Build history of the part. All positions in model axes, mm. Round coordinates to 2 decimals unless told otherwise and drop trailing zeros. Loops run counter-clockwise (first coordinate to the right, second up) from the corner with the lowest first, then second, coordinate; pieces in that order, holes last. Notation, with made-up numbers: (22.5, -0.75) - (33.5, -0.75) arc R29 ccw to (33.5, 31.25) - close; hole circle Ø10 at (0, 82.5). An arc over 180 degrees is marked (long way). Use one line per item in the form item = value. Start each with the question number.
Q1. Saw through at C-C (y = 8.5). Give the cut face in (x, z).
Q2. Saw through at D-D (z = -13). Give the cut face in (x, y).
Q3. Saw through at A-A (z = 0). Give the cut face in (x, y).
Q4. Pin check, flat tips, straight feed: pin 1 (1.4 mm diameter, centred on x = -2, z = 13, fed in from -Y); pin 2 (1.5 mm diameter, centred on x = -1, y = 42, fed in from +Z); pin 3 (1.5 mm diameter, centred on x = -2, z = -10, fed in from +Y). Stop position of each tip, or through.
Q5. Drill centre lines: line 1 (Z direction, x = -2.25, y = 0); line 2 (Y direction, x = -2.3, z = -0.5); line 3 (Y direction, x = -0.8, z = -4.75). Where is each one in solid material? Low to high.
Q6. Saw through at B-B (x = -0.5). Give the cut face in (y, z), then the cut area to 3 significant figures.
```python
from build123d import *

# Parameters (mm, degrees)
ESQUISSE1_R        = 10.75
BOSS_EXTRU_1_DEPTH = 3


with BuildPart() as part:
    # Esquisse1 → Boss.-Extru.1 (new body)
    with BuildSketch(Plane(origin=(-3, 0, 0), x_dir=(0, -1, 0), z_dir=(-1, 0, 0))):
        Polygon((40, 15), (-40, 15), (-40, 12.2), (-43, 12.2), (-43, -7.8), (-40, -7.8), (-40, -15), (40, -15), (40, -7.8), (43, -7.8), (43, 12.2), (40, 12.2), align=None)
        with Locations(Location((0, 0, 0), (0, 0, 180))):
            Circle(ESQUISSE1_R, mode=Mode.SUBTRACT)
    extrude(amount=-BOSS_EXTRU_1_DEPTH)


solid = part.part
```
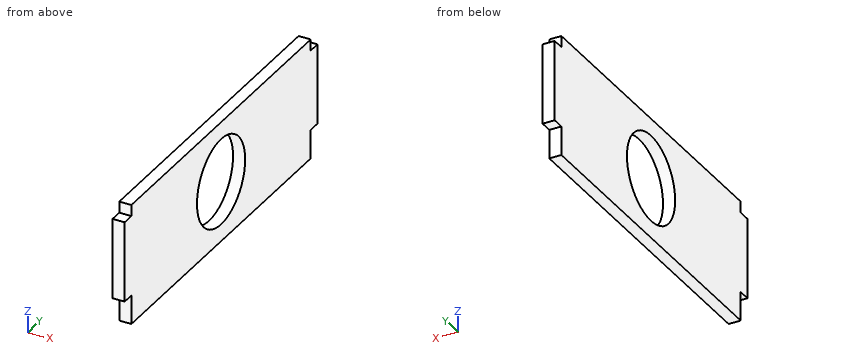
Report:
q1.outline = (-3, -15) - (0, -15) - (0, -6.58) - (-3, -6.58) - close; (-3, 6.58) - (0, 6.58) - (0, 15) - (-3, 15) - close
q2.outline = (-3, -40) - (0, -40) - (0, 40) - (-3, 40) - close
q3.outline = (-3, -43) - (0, -43) - (0, -10.75) - (-3, -10.75) - close; (-3, 10.75) - (0, 10.75) - (0, 43) - (-3, 43) - close
q4.pin_1 = -40
q4.pin_2 = 12.2
q4.pin_3 = 40
q5.line_1 = -15 to -10.75, 10.75 to 15
q5.line_2 = -43 to -10.74, 10.74 to 43
q5.line_3 = -43 to -9.64, 9.64 to 43
q6.outline = (-43, -7.8) - (-40, -7.8) - (-40, -15) - (40, -15) - (40, -7.8) - (43, -7.8) - (43, 12.2) - (40, 12.2) - (40, 15) - (-40, 15) - (-40, 12.2) - (-43, 12.2) - close; hole circle Ø21.5 at (0, 0)
q6.area = 2,160 mm²
